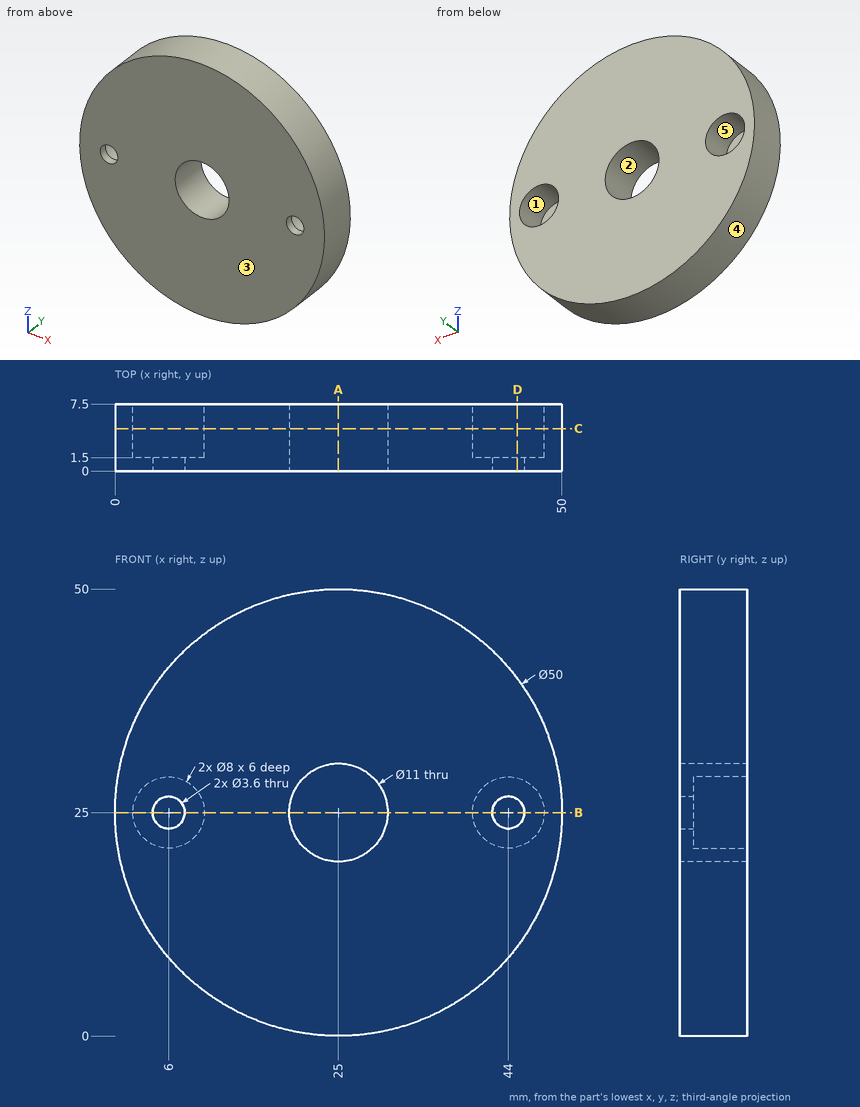
Input: dimensioned drawing with shaded views. Units: mm. Origin: part minimum x, y, z. A direction names the side the tool comes from. Coordinates: 2 decimals unless noted, no trailing zeros. Write each loop counter-clockwise with the first axis right and the second up, starting at its lowest first coordinate (ties: lowest second). Pieces come first, ordered by that corner, then holes. Notation, with made-up numbers: M 4,82.5 L 59,82.5 A32 ccw 59,114.5 Z; hole C 71,45 d8. An arc over 180 degrees is marked long. Answer as a JSON object with one key per item and string values. Group by question number.
(1) Section B-B on z = 25. Output: boundary loops of the cut face in (x, y), plus the area to 3 significant figures.
(2) Set-up query: the marked faces 1 and 2. Return all of +Z, -Z, +X, -X, +Y, -Y with unobstructed straight access to the full face (end or side cutting, diameter ignored); none if empty.
(3) Section A-A on x = 25. Output: boundary loops of the cut face in (y, z).
(4) Mould query, pull axis X, two halves, no side actions, for the marked faces 3, 4 and 5. Classes: pulls with the +X half, pulls with the -X half, needs draft (parallel to the pull), parting line crosses it, or undercut.
(5) Contact query for flat-ended pins moving along their axis: P1, Ø7, axis at x = 6, z = 25, coming from the +Y side; P2, Ø1, axis at x = 15.5, y = 2, coming from the -Z side; P3, Ø1, axis at x = 36.5, y = 6.5, coming from the +Z side; P4, Ø2, axis at x = 44, z = 25, coming from the -Y side. Output: stop coordinate, or through.
(6) Section D-D on x = 45. Output: boundary loops of the cut face in (y, z).
(7) Ray query, line 1 along X through (y, z) = (1.75, 25); line 2 along X through (y, z) = (1.15, 25); line 3 along Y through (x, z) = (42, 22). Return the intervals inside material, ascending. Write a range as [from, to].
(8) Section C-C on y = 4.75. Output: boundary loops of the cut face in (x, z), plus the area to 3 significant figures.
Result set:
{
 "1": {"outline": "M 0,0 L 4.2,0 L 4.2,1.5 L 2,1.5 L 2,7.5 L 0,7.5 Z; M 7.8,0 L 19.5,0 L 19.5,7.5 L 10,7.5 L 10,1.5 L 7.8,1.5 Z; M 30.5,0 L 42.2,0 L 42.2,1.5 L 40,1.5 L 40,7.5 L 30.5,7.5 Z; M 45.8,0 L 50,0 L 50,7.5 L 48,7.5 L 48,1.5 L 45.8,1.5 Z", "area": "186 mm2"},
 "2": {"face 1": "+Y", "face 2": "+Y, -Y"},
 "3": {"outline": "M 0,0 L 7.5,0 L 7.5,19.5 L 0,19.5 Z; M 0,30.5 L 7.5,30.5 L 7.5,50 L 0,50 Z"},
 "4": {"face 3": "needs draft", "face 4": "parting line crosses it", "face 5": "undercut"},
 "5": {"P1": "stops at y = 1.5", "P2": "stops at z = 1.68", "P3": "stops at z = 47.45", "P4": "passes through"},
 "6": {"outline": "M 0,10 L 7.5,10 L 7.5,21.13 L 1.5,21.13 L 1.5,23.5 L 0,23.5 Z; M 0,26.5 L 1.5,26.5 L 1.5,28.87 L 7.5,28.87 L 7.5,40 L 0,40 Z"},
 "7": {"line 1": "x = [0, 2], [10, 19.5], [30.5, 40], [48, 50]", "line 2": "x = [0, 4.2], [7.8, 19.5], [30.5, 42.2], [45.8, 50]", "line 3": "y = [0, 1.5]"},
 "8": {"outline": "C 25,25 d50; hole C 6,25 d8; hole C 25,25 d11; hole C 44,25 d8", "area": "1,770 mm2"}
}
